The model under review builds one solid part; all positions refer to its coordinate system, in mm. Face numbers are marked on the shaded views. Round coordinates to 2 decimals unless told otherwise and drop trailing zeros. Loops run counter-clockwise (first coordinate to the right, second up) from the corner with the lowest first, then second, coordinate; pieces in that order, holes last. Notation, with made-up numbers: (81.25, 54) -> (129.25, 54) arc R31 cw to (129.25, 88) -> close; hole circle Ø1 at (4.5, -27). An arc over 180 degrees is marked (long way). Write each question's results on one line, items separated by ' | '. Start each with the question number.
Item 1: We need section A-A (z = 13). Give the boundary of the cut face in (x, y).
Item 2: We need section B-B (x = -2). Give the boundary of the cut face in (y, z).
Item 3: We need section D-D (x = 4.5). Give the boundary of the cut face in (y, z), and give its area (3 significant figures).
Item 4: For L1, parallel to X at y = 1.2, z = 24; L2, parallel to Z at x = 5, y = 1.3; L3, parallel to Z at x = 3, y = 1.45, list the stretches that pass through material, from the lowest coordinate up. Write a range as from..to.
Item 5: We need section C-C (y = 2.55). Give the boundary of the cut face in (x, z), and give its area (3 significant figures).
Item 6: Mouldability with a two-part tool opening along X and no side actions: class the marked faces 1, 2, 3 and 4 as pulls with the +X half, pulls with the -X half, needs draft (parallel to the pull), parting line crosses it, or undercut.
Item 7: Clearance check with a flat-ended pin moving along its axis: pin 1 Ø3 at (x, z) = (-1.5, 12) entering from -Y. State where the tip first meets the part, or that it passes through.
from build123d import *

# Parameters (mm, degrees)
EXTRUDE_1_DEPTH          = 26.5
EXTRUDE_1_DEPTH_BACK     = 3.5
CUT_EXTRUDE_1_DEPTH      = 28.950313057
CUT_EXTRUDE_1_DEPTH_BACK = 28.950313057
SKETCH_3_W               = 14.8
SKETCH_3_H               = 28
CUT_EXTRUDE_2_DEPTH      = 1
CHAMFER_1_SIZE           = 0.5
CHAMFER_2_SIZE           = 0.5


with BuildPart() as part:
    # Эскиз1 → Бобышка-Вытянуть1 (new, two sides: drawn at the far end of the back side and taken through both)
    with BuildSketch(Plane.XY.offset(-EXTRUDE_1_DEPTH_BACK)):
        Polygon((-2.439262184, 0.9), (2.439262184, 0.9), (8.4, 0.9), (8.4, 1.8), (8.4, 1.82), (3, 2.9), (-3, 2.9), (-8.4, 1.82), (-8.4, 1.8), (-8.4, 0.9), align=None)
    extrude(amount=EXTRUDE_1_DEPTH + EXTRUDE_1_DEPTH_BACK)

    # Эскиз2 → Вырез-Вытянуть1 (cut, two sides: drawn at the far end of the back side and taken through both)
    with BuildSketch(Plane(origin=(0, 0, 0), x_dir=(0, 0, -1), z_dir=(1, 0, 0)).offset(-CUT_EXTRUDE_1_DEPTH_BACK)):
        Polygon((-25.5, 2.9), (-26.5, 2.9), (-26.5, 2.2), align=None)
    extrude(amount=CUT_EXTRUDE_1_DEPTH + CUT_EXTRUDE_1_DEPTH_BACK, mode=Mode.SUBTRACT)

    # Эскиз3 → Вырез-Вытянуть2 (cut)
    with BuildSketch(Plane.XZ.offset(-0.9)):
        with Locations((0, 11.5)):
            Rectangle(SKETCH_3_W, SKETCH_3_H)
    extrude(amount=-CUT_EXTRUDE_2_DEPTH, mode=Mode.SUBTRACT)

    # Фаска1
    chamfer_1_edges = [part.edges().sort_by_distance(p)[0] for p in [
        (-7.4, 1.9, 11.5),
        (0, 1.9, 25.5),
        (7.4, 1.9, 11.5),
        (0, 1.9, -2.5),
    ]]
    chamfer(chamfer_1_edges, length=CHAMFER_1_SIZE)

    # Фаска2
    chamfer_2_edges = [part.edges().sort_by_distance(p)[0] for p in [
        (8.4, 1.36, 26.5),
        (-8.4, 1.36, 26.5),
        (-8.4, 1.36, -3.5),
        (8.4, 1.36, -3.5),
    ]]
    chamfer(chamfer_2_edges, length=CHAMFER_2_SIZE)


solid = part.part
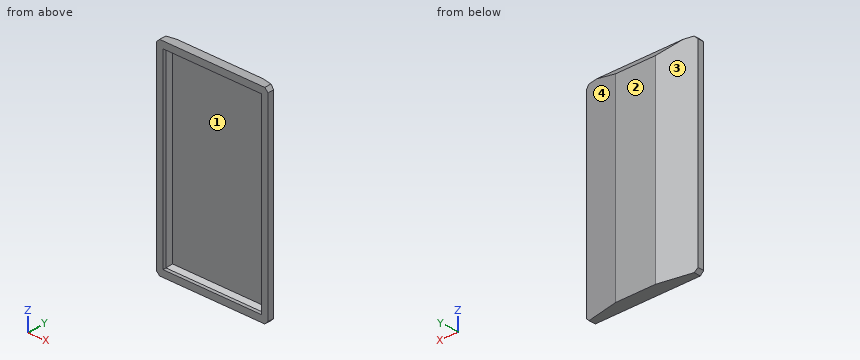
Here are the results:
1) outline: (-8.4, 0.9) -> (-7.4, 0.9) -> (-7.4, 1.4) -> (-6.9, 1.9) -> (6.9, 1.9) -> (7.4, 1.4) -> (7.4, 0.9) -> (8.4, 0.9) -> (8.4, 1.82) -> (3, 2.9) -> (-3, 2.9) -> (-8.4, 1.82) -> close
2) outline: (0.9, -3.5) -> (2.9, -3.5) -> (2.9, 25.5) -> (2.2, 26.5) -> (0.9, 26.5) -> (0.9, 25.5) -> (1.4, 25.5) -> (1.9, 25) -> (1.9, -2) -> (1.4, -2.5) -> (0.9, -2.5) -> close
3) outline: (0.9, -3.5) -> (2.6, -3.5) -> (2.6, 25.93) -> (2.2, 26.5) -> (0.9, 26.5) -> (0.9, 25.5) -> (1.4, 25.5) -> (1.9, 25) -> (1.9, -2) -> (1.4, -2.5) -> (0.9, -2.5) -> close | area: 23.1 mm2
4) L1: x = -8.4..-7.4, 7.4..8.4 | L2: z = -3.5..-2.5, 25.5..26.5 | L3: z = -3.5..-2.45, 25.45..26.5
5) outline: (-4.75, -3.5) -> (4.75, -3.5) -> (4.75, 26) -> (-4.75, 26) -> close | area: 280 mm2
6) face 1: undercut | face 2: needs draft | face 3: pulls with the -X half | face 4: pulls with the +X half
7) pin 1: stops at y = 1.9
